```python
from build123d import *

# Parameters (mm, degrees)
SKETCH_1_R          = 5
EXTRUDE_1_DEPTH     = 35
SKETCH_2_R          = 2.5
CUT_EXTRUDE_1_DEPTH = 48.968739821


with BuildPart() as part:
    # Эскиз1 → Бобышка-Вытянуть1 (new body)
    with BuildSketch(Plane.XY):
        Polygon((-18.5, 21), (-10, 21), (-7.5, 26), (7.5, 26), (10, 21), (18.5, 21), (18.5, 12), (20, 8), (20, 0), (5, 0), (5, 1.5), (-5, 1.5), (-5, 0), (-20, 0), (-20, 8), (-18.5, 12), align=None)
        with Locations((0, 13)):
            Circle(SKETCH_1_R, mode=Mode.SUBTRACT)
    extrude(amount=EXTRUDE_1_DEPTH)

    # Эскиз2 → Вырез-Вытянуть1 (cut, through all)
    with BuildSketch(Plane.XZ):
        with Locations(Location((-14, 28, 0), (0, 0, 270))):
            Circle(SKETCH_2_R)
        with Locations(Location((14, 28, 0), (0, 0, 270))):
            Circle(SKETCH_2_R)
        with Locations(Location((14, 7, 0), (0, 0, 270))):
            Circle(SKETCH_2_R)
        with Locations(Location((-14, 7, 0), (0, 0, 270))):
            Circle(SKETCH_2_R)
    extrude(amount=-CUT_EXTRUDE_1_DEPTH, mode=Mode.SUBTRACT)


solid = part.part
```
Check sheet for the modelled part. Datum: model origin and axes. Units: mm. A direction names the side the tool comes from. Give positions to 0.01 mm unless a question says otherwise; leave off trailing zeros. Write each loop counter-clockwise with the first axis right and the second up, starting at its lowest first coordinate (ties: lowest second). Pieces come first, ordered by that corner, then holes. Notation, with made-up numbers: (-24.5, -37) -> (24.5, -37) arc R16 ccw to (24.5, -25) -> close; hole circle Ø4 at (-23, -21.75). An arc over 180 degrees is marked (long way). Use CSV: the item, a comma, the result in double quotes. Start each with the question number.
Q1. Cross-section at B-B on z = 28. Enter the section's corners in (x, y).
Q2. Depth check by flat-ended pin: P1, Ø5, axis at y = 20, z = 22, coming from the -X side; P2, Ø6, axis at y = 13, z = 26, coming from the -X side; P3, Ø2.5, axis at x = 13, z = 24.5, coming from the +Y side. Enter the tip coordinate at first touch or a pass-through.
Q3. Cross-section at C-C on y = 5.5. Enter the section's corners in (x, z).
Q4. Cross-section at D-D on x = 0. Enter the section's corners in (y, z).
Q5. Tool access check on faces 1 (the flat face through (0, 7, 0)), 2 (the flat face through (14, 21, 17)), 3 (the flat face through (-5, 1, 17)). Record the directions out of +Z, -Z, +X, -X, +Y, -Y that give a thin tool (end or side, any length) a straight path to the whole face; none if there is none.
Q6. Scan lines: line 1 along X through (y, z) = (4.5, 7); line 2 along X through (y, z) = (13.25, 7); line 3 along Y through (x, z) = (0, 23.5). Record each from-to range of solid material in increasing order.
Q7. Cross-section at A-A on y = 13. Enter the section's corners in (x, z), and give its area (3 significant figures).
Q8. Release check for a two-part mould opening along X. For faces 4 (the flat face through (-14, 21, 17)), 5 (the cylindrical face through (-0.651, 17.957, 17.255)), 6 (the flat face through (0, 1.5, 17)), 7 (the flat face through (20, 4, 17)) record: +X half, -X half, draft (parallel to the pull), parting line (faces both ways), or undercut.
Working result:
1,outline,"(-20, 0) -> (-16.5, 0) -> (-16.5, 21) -> (-18.5, 21) -> (-18.5, 12) -> (-20, 8) -> close; (-11.5, 0) -> (-5, 0) -> (-5, 1.5) -> (5, 1.5) -> (5, 0) -> (11.5, 0) -> (11.5, 21) -> (10, 21) -> (7.5, 26) -> (-7.5, 26) -> (-10, 21) -> (-11.5, 21) -> close; (16.5, 0) -> (20, 0) -> (20, 8) -> (18.5, 12) -> (18.5, 21) -> (16.5, 21) -> close; hole circle Ø10 at (0, 13)"
2,P1,"stops at x = -18.5"
2,P2,"stops at x = -19.25"
2,P3,"stops at y = 21"
3,outline,"(-20, 0) -> (20, 0) -> (20, 35) -> (-20, 35) -> close; hole circle Ø5 at (-14, 7); hole circle Ø5 at (-14, 28); hole circle Ø5 at (14, 7); hole circle Ø5 at (14, 28)"
4,outline,"(1.5, 0) -> (8, 0) -> (8, 35) -> (1.5, 35) -> close; (18, 0) -> (26, 0) -> (26, 35) -> (18, 35) -> close"
5,face 1,"-Z, +X, -X, +Y, -Y"
5,face 2,"+Z, -Z, +X, +Y"
5,face 3,"+Z, -Z, -Y"
6,line 1,"x = -20 to -16.5, -11.5 to 11.5, 16.5 to 20"
6,line 2,"x = -18.5 to -16.5, -11.5 to -4.99, 4.99 to 11.5, 16.5 to 18.5"
6,line 3,"y = 1.5 to 8, 18 to 26"
7,outline,"(-18.5, 0) -> (-5, 0) -> (-5, 35) -> (-18.5, 35) -> close; (5, 0) -> (18.5, 0) -> (18.5, 35) -> (5, 35) -> close; hole circle Ø5 at (-14, 7); hole circle Ø5 at (-14, 28); hole circle Ø5 at (14, 7); hole circle Ø5 at (14, 28)"
7,area,"866 mm^2"
8,face 4,"draft"
8,face 5,"undercut"
8,face 6,"undercut"
8,face 7,"+X half"
